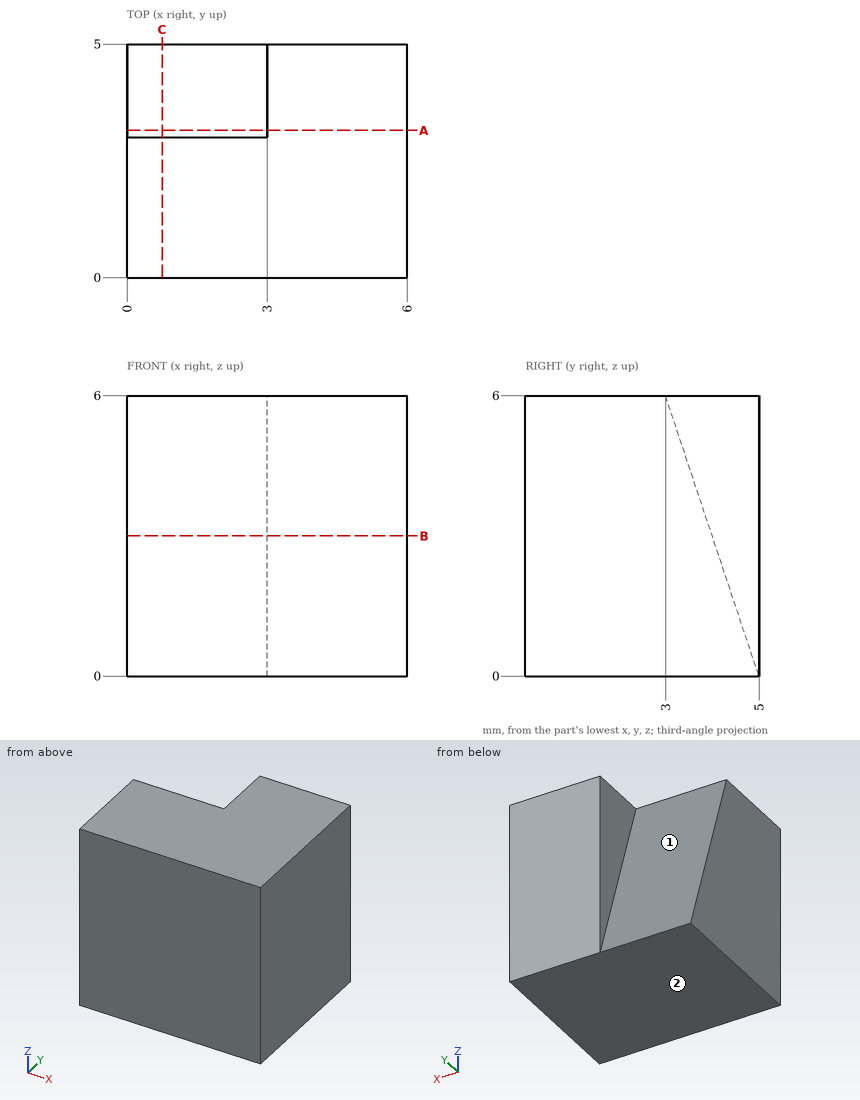
Geometry check sheet. Reference: drawing and pictorial views, mm from the part's lowest x, y, z. A direction names the side the tool comes from. Coordinates: 2 decimals unless noted, no trailing zeros. Order: outer loops, then holes, each group sorted by start corner. A loop starts at its lowest first (then second) coordinate and runs counter-clockwise, first axis right, second up.
Item 1: Section check B-B, the plane z = 3. Enter the section's corners in (x, y).
Filled in:
outline: (0, 0) - (6, 0) - (6, 5) - (3, 5) - (3, 4) - (0, 4) - close
Item 2: Material ranges on L1, parallel to X at y = 3.4, z = 5.75; L2, parallel to Y at x = 2.05, z = 2; L3, parallel to Y at x = 2.65, z = 2.25, recorded low to high.
Filled in:
L1: x = 3 to 6
L2: y = 0 to 4.33
L3: y = 0 to 4.25
Item 3: Section check C-C, the plane x = 0.75. Enter the section's corners in (y, z).
Filled in:
outline: (0, 0) - (5, 0) - (3, 6) - (0, 6) - close
Item 4: Section check A-A, the plane y = 3.15. Enter the section's corners in (x, z), then the cut area to 4 significant figures.
Filled in:
outline: (0, 0) - (6, 0) - (6, 6) - (3, 6) - (3, 5.55) - (0, 5.55) - close
area: 34.65 mm2
Item 5: Access from +Z, -Z, +X, -X, +Y, -Y to the whole of each face (thin tool, end or side, straight path). Record for the marked faces 1 and 2.
Filled in:
face 1: +Z, -X, +Y
face 2: -Z, +X, -X, +Y, -Y
